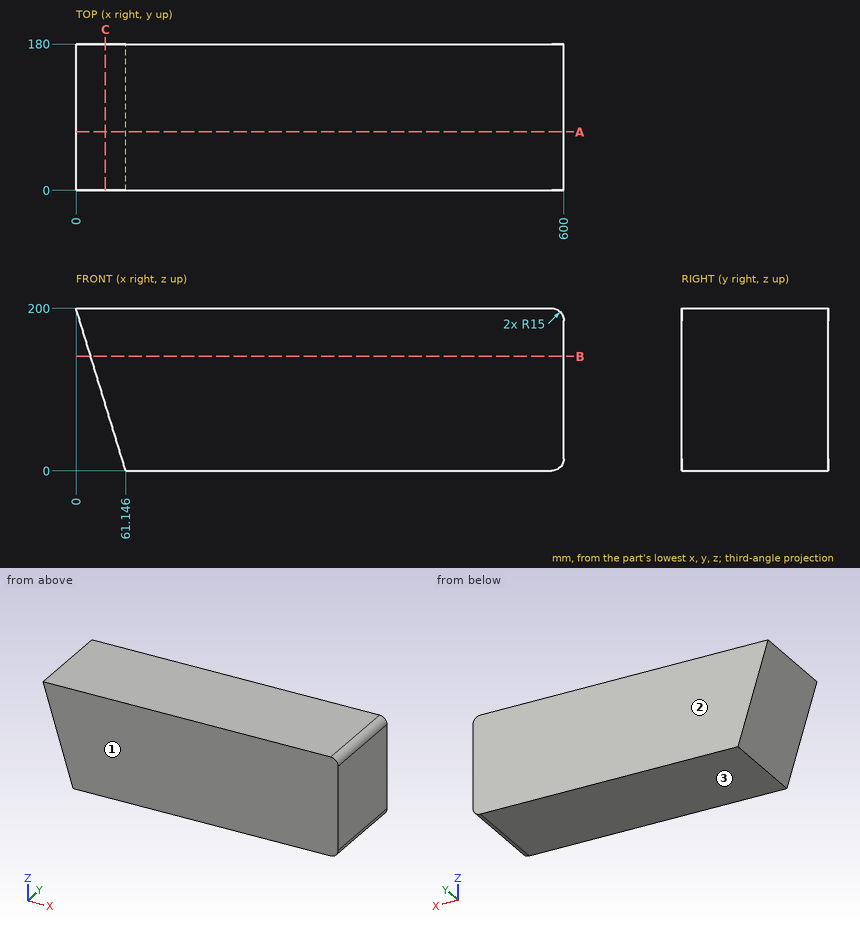
Input: dimensioned drawing with shaded views. Units: mm. Origin: part minimum x, y, z. Give positions to 0.01 mm unless a question says otherwise; leave off trailing zeros. Order: outer loops, then holes, each group sorted by start corner. A loop starts at its lowest first (then second) coordinate and runs counter-clockwise, first axis right, second up. Notation, with made-up numbers: (-21.5, -8.5) -> (-5.5, -8.5) arc R29 cw to (-5.5, 14.5) -> close; hole circle Ø3 at (-24, 13). An arc over 180 degrees is marked (long way). Write item = value, one per line.
Item 1: Section query B-B (z = 141). Output: boundary loops of the cut face in (x, y), then the cut area to 3 significant figures.
Check result:
outline = (18.04, 0) -> (600, 0) -> (600, 180) -> (18.04, 180) -> close
area = 105,000 mm²
Item 2: Mould query, pull axis Y, two halves, no side actions, for the marked faces 1, 2 and 3. Classes: +Y half, -Y half, draft (parallel to the pull), parting line (faces both ways), or undercut.
Check result:
face_1 = -Y half
face_2 = +Y half
face_3 = draft
Item 3: Contact query for flat-ended pins moving along their axis: pin 1 (1.5 mm diameter, centred on y = 46, z = 166, fed in from -X); pin 2 (12 mm diameter, centred on y = 136.5, z = 133.5, fed in from -X); pin 3 (5 mm diameter, centred on y = 159, z = 25.5, fed in from -X). Output: stop coordinate, or through.
Check result:
pin_1 = 10.17
pin_2 = 18.5
pin_3 = 52.59
Item 4: Ray query, probe 1 along X at (y, z) = (131.5, 156.5); probe 2 along X at (y, z) = (55, 98). Return the intervals inside material, ascending.
Check result:
probe_1 = 13.3 to 600
probe_2 = 31.18 to 600
Item 5: Section query A-A (y = 72). Output: boundary loops of the cut face in (x, z), then the cut area to 3 significant figures.
Check result:
outline = (0, 200) -> (61.15, 0) -> (585, 0) arc R15 ccw to (600, 15) -> (600, 185) arc R15 ccw to (585, 200) -> close
area = 114,000 mm²
Item 6: Section query C-C (x = 36). Output: boundary loops of the cut face in (y, z).
Check result:
outline = (0, 82.25) -> (180, 82.25) -> (180, 200) -> (0, 200) -> close
